Print and shaded views of the part. All mm, measured from the part's lowest x, y and z. A direction names the side the tool comes from. Coordinates: 2 decimals unless noted, no trailing zeros. Order: outer loops, then holes, each group sorted by start corner. A loop starts at its lowest first (then second) coordinate and runs counter-clockwise, first axis right, second up. Notation, with made-up numbers: M 71,-18 L 90,-18 A10 ccw 90,-8 Z; hole C 68,78 d8. An arc over 180 degrees is marked long. Use a Markdown table: item, result. Add a question column.
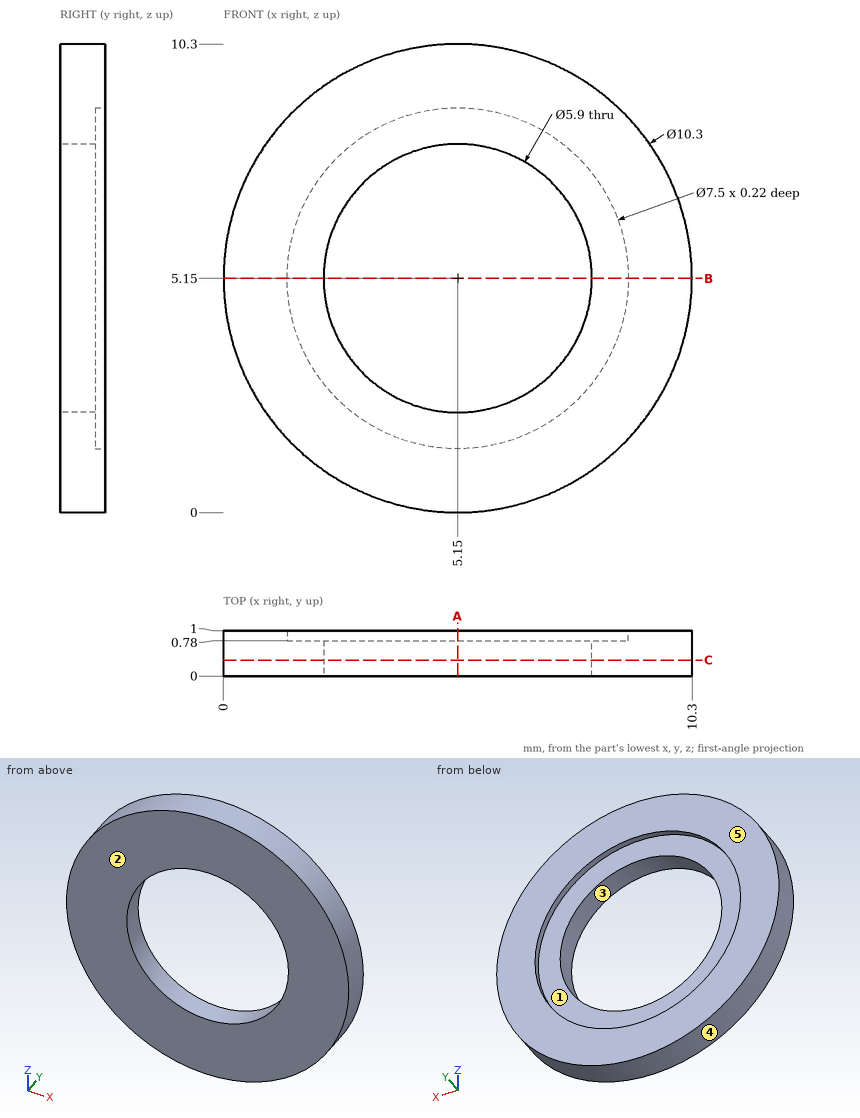
(1) Slice it at A-A on x = 5.15. Give the cut face in (y, z).
(2) Which spindle directions (+Z, -Z, +X, -X, +Y, -Y) get a long thin tool onto all of the face, cutting with end or side? Do the marked faces 1 and 2. Say none if no direction does.
(3) Slice it at B-B on z = 5.15. Give the cut face in (x, y).
(4) Slice it at C-C on y = 0.35. Give the cut face in (x, z), and give its area (3 significant figures).
(5) Drill centre lines: line 1 along Z through (x, y) = (5.15, 0.3); line 2 along Z through (x, y) = (5.15, 0.95); line 3 along Y through (x, z) = (3, 7.5). Where is each one in solid material? Low to high. Write a range as from..to.
(6) Mould opens along X. For the marked faces 3, 4 and 5 say: released by +X, released by -X, zero draft, split by the parting line, or undercut.
Solutions:
| question | item | result |
|---|---|---|
| 1 | outline | M 0,0 L 1,0 L 1,1.4 L 0.78,1.4 L 0.78,2.2 L 0,2.2 Z; M 0,8.1 L 0.78,8.1 L 0.78,8.9 L 1,8.9 L 1,10.3 L 0,10.3 Z |
| 2 | face 1 | +Y |
| 2 | face 2 | +Z, -Z, +X, -X, -Y |
| 3 | outline | M 0,0 L 2.2,0 L 2.2,0.78 L 1.4,0.78 L 1.4,1 L 0,1 Z; M 8.1,0 L 10.3,0 L 10.3,1 L 8.9,1 L 8.9,0.78 L 8.1,0.78 Z |
| 4 | outline | C 5.15,5.15 d10.3; hole C 5.15,5.15 d5.9 |
| 4 | area | 56.0 mm² |
| 5 | line 1 | 0..2.2, 8.1..10.3 |
| 5 | line 2 | 0..1.4, 8.9..10.3 |
| 5 | line 3 | 0..0.78 |
| 6 | face 3 | undercut |
| 6 | face 4 | split by the parting line |
| 6 | face 5 | zero draft |
